```python
from build123d import *

# Parameters (mm, degrees)
CYLINDER002001007_R     = 2
CYLINDER002001007_DEPTH = 23.3333
ARRAY001_X_COUNT        = 2
ARRAY001_X_PITCH        = 34
ARRAY001_Y_COUNT        = 2
ARRAY001_Y_PITCH        = 30
CYLINDER002001006_R     = 26.6667
CYLINDER002001006_DEPTH = 3


with BuildPart() as obj1:
    # Cylinder002001007 → Cylinder002001007 (new body)
    with BuildSketch(Plane(origin=(25, 150, 0), x_dir=(1, 0, 0), z_dir=(0, 0, 1))):
        Circle(CYLINDER002001007_R)
    extrude(amount=CYLINDER002001007_DEPTH)

    # Array001 X: obj1_2


with BuildPart() as obj1_1:
    add(obj1.part)
    with Locations(*[(i * ARRAY001_X_PITCH, 0, 0) for i in range(1, ARRAY001_X_COUNT)]):
        add(obj1.part)

    # Array001 Y: obj1_2


with BuildPart() as obj1_2:
    add(obj1_1.part)
    with Locations(*[(0, i * ARRAY001_Y_PITCH, 0) for i in range(1, ARRAY001_Y_COUNT)]):
        add(obj1_1.part)


with BuildPart() as obj2:
    # Cylinder002001006 → Cylinder002001006 (new body)
    with BuildSketch(Plane(origin=(42, 165, 23.3333), x_dir=(1, 0, 0), z_dir=(0, 0, 1))):
        Circle(CYLINDER002001006_R)
    extrude(amount=CYLINDER002001006_DEPTH)

    # Fusion010: union obj1
    add(obj1_2.part)


solid = obj2.part
```
The listing builds one solid part. Answer for the finished solid, in the listing's coordinates (mm). A direction names the side the tool comes from. Round coordinates to 2 decimals unless told otherwise and drop trailing zeros. Loops run counter-clockwise (first coordinate to the right, second up) from the corner with the lowest first, then second, coordinate; pieces in that order, holes last.
Q1. Section B-B, the plane x = 59 is taken. Determine the outline of the cut face in (y, z).
Q2. Section C-C, the plane y = 165 is taken. Determine the outline of the cut face in (x, z).
Q3. Section A-A, the plane z = 12 is taken. Determine the outline of the cut face in (x, y).
Q4. For a pull along Y with two mould halves and no side action, classify faces 3 (the face through (42, 165, 26.333)), 4 (the face through (66.633, 154.786, 24.812)), 5 (the face through (25.923, 178.226, 11.503)) as released by +Y, released by -Y, zero draft, split by the parting line, or undercut.
Q5. Which of the six approach directions +Z, -Z, +X, -X, +Y, -Y give full straight-line access (tool end or side, diameter ignored) to faces 1 (the face through (25, 150, 0)), 2 (the face through (25.923, 148.226, 11.503))?
Q6. Find the intervals of material crossed by line 1 (Z direction, x = 33, y = 162); line 2 (X direction, y = 149.5, z = 12.25); line 3 (Y direction, x = 58, z = 15.75), in increasing order.
Q7. Section D-D, the plane y = 150 is taken. Determine the outline of the cut face in (x, z), then the cut area to 3 significant figures.
Q8. Given pin 1 Ø8 at (x, z) = (26, 4.5) entering from +Y; pin 2 Ø3 at (y, z) = (179, 21.5) entering from -X; pin 3 Ø4 at (x, z) = (30.5, 17) entering from +Y; pin 4 Ø6 at (y, z) = (148, 18) entering from +X, each flat-ended and moving along its own axis, determine where each tip first touches the part or whether it passes through.
Completed:
1. outline: (144.45, 23.33) - (148, 23.33) - (148, 0) - (152, 0) - (152, 23.33) - (178, 23.33) - (178, 0) - (182, 0) - (182, 23.33) - (185.55, 23.33) - (185.55, 26.33) - (144.45, 26.33) - close
2. outline: (15.33, 23.33) - (68.67, 23.33) - (68.67, 26.33) - (15.33, 26.33) - close
3. outline: circle Ø4 at (25, 150); circle Ø4 at (25, 180); circle Ø4 at (59, 150); circle Ø4 at (59, 180)
4. face 3: zero draft
4. face 4: split by the parting line
4. face 5: undercut
5. face 1: -Z, +X, -X, +Y, -Y
5. face 2: -Z
6. line 1: z = 23.33 to 26.33
6. line 2: x = 23.06 to 26.94, 57.06 to 60.94
6. line 3: y = 148.27 to 151.73, 178.27 to 181.73
7. outline: (19.95, 23.33) - (23, 23.33) - (23, 0) - (27, 0) - (27, 23.33) - (57, 23.33) - (57, 0) - (61, 0) - (61, 23.33) - (64.05, 23.33) - (64.05, 26.33) - (19.95, 26.33) - close
7. area: 319 mm2
8. pin 1: stops at y = 182
8. pin 2: stops at x = 23
8. pin 3: passes through
8. pin 4: stops at x = 61
